Geometry check sheet. Reference: the model listing, model coordinates, mm. A direction names the side the tool comes from. Give positions to 0.01 mm unless a question says otherwise; leave off trailing zeros. Loops run counter-clockwise (first coordinate to the right, second up) from the corner with the lowest first, then second, coordinate; pieces in that order, holes last. Notation, with made-up numbers: (19, 64) - (44, 64) arc R14 cw to (44, 82) - close; hole circle Ø11 at (61.5, 11). An arc over 180 degrees is marked (long way). Use a Markdown table: item, result. Add a question column.
1. Material ranges on L1, parallel to Y at x = -11, z = 24; L2, parallel to Y at x = 30, z = -16; L3, parallel to Z at x = 6.5, y = 6, recorded low to high.
2. Cross-section at C-C on y = 31. Enter the section's corners in (x, z).
3. Cross-section at A-A on y = -19. Enter the section's corners in (x, z), and give its area (3 significant figures).
4. Draft check along X on faces 1 (the flat face through (0, -15, -15)), 2 (the flat face through (0, -50, 0)), 3 (the flat face through (-30, 49, 0)). Enter one of: pulls with the +X half, pulls with the -X half, needs draft (parallel to the pull), parting line crosses it, or undercut.
5. Depth check by flat-ended pin: P1, Ø11, axis at x = 4, z = -23.5, coming from the +Y side; P2, Ø16, axis at y = -9, z = -22, coming from the -X side; P3, Ø8, axis at x = 35.5, z = 39, coming from the -Y side. Enter the tip coordinate at first touch or a pass-through.
6. Cross-section at B-B on x = 0. Enter the section's corners in (y, z), and give its area (3 significant figures).
7. Set-up check for faces 4 (the flat face through (30, 49, 0)), 5 (the flat face through (0, 0, 16)), 6 (the flat face through (0, 49, -7.5)), 7 (the flat face through (5, -15, -22)): record each of +Z, -Z, +X, -X, +Y, -Y from which the full face is reachable in a straight line by a thin tool's end or side.
from build123d import *

# Parameters (mm, degrees)
F0_W     = 60
F0_H     = 15
F1_DEPTH = 100
F3_DEPTH = 30
F4_R     = 50
F4_R_2   = 30
F5_DEPTH = 20
F6_R     = 15
F8_DEPTH = 30


# Not quite as in the source:
# - a feature names something its author has since deleted; it is built from what else it names


with BuildPart() as f1:
    # F0 (on Front) → F1 (new body)
    with BuildSketch(Plane.XZ):
        Rectangle(F0_W, F0_H)
    extrude(amount=-F1_DEPTH)

    # F2 (on face) → F3 (join)
    with BuildSketch(Plane.XZ):
        with BuildLine():
            ThreePointArc((29.0473750966, -7.5), (29.760890888, -3.7801287745), (30, 0))
            ThreePointArc((30, 0), (29.760890888, 3.7801287745), (29.0473750966, 7.5))
            Line((29.0473750966, 7.5), (-29.0473750966, 7.5))
            ThreePointArc((-29.0473750966, 7.5), (-29.760890888, 3.7801287745), (-30, 0))
            ThreePointArc((-30, 0), (-29.760890888, -3.7801287745), (-29.0473750966, -7.5))
            Line((-29.0473750966, -7.5), (29.0473750966, -7.5))
        make_face()
        with BuildLine():
            Line((-29.0473750966, 7.5), (29.0473750966, 7.5))
            ThreePointArc((29.0473750966, 7.5), (0, 30), (-29.0473750966, 7.5))
        make_face()
        with BuildLine():
            ThreePointArc((-29.0473750966, -7.5), (0, -30), (29.0473750966, -7.5))
            Line((29.0473750966, -7.5), (-29.0473750966, -7.5))
        make_face()
    extrude(amount=F3_DEPTH)

    # F4 (on face) → F5 (join)
    with BuildSketch(Plane.XZ.offset(30)):
        Circle(F4_R)
        Circle(F4_R_2, mode=Mode.SUBTRACT)
        Circle(F4_R_2)
    extrude(amount=F5_DEPTH)

    # F6
    f6_edges = [f1.edges().sort_by_distance(p)[0] for p in [
        (-50, -50, 0),
    ]]
    fillet(f6_edges, radius=F6_R)

    # F7 (on face) → F8 (cut)
    with BuildSketch(Plane(origin=(0, 0, 0), x_dir=(-1, 0, 0), z_dir=(0, 1, 0))):
        with BuildLine():
            Line((5, -15), (-5, -15))
            Line((-5, -15), (-5, -29.5803989155))
            ThreePointArc((-5, -29.5803989155), (0, -30), (5, -29.5803989155))
            Line((5, -29.5803989155), (5, -15))
        make_face()
    extrude(amount=-F8_DEPTH, mode=Mode.SUBTRACT)


solid = f1.part
Values found:
| question | item | result |
|---|---|---|
| 1 | L1 | y = -50 to 0 |
| 1 | L2 | y = -50 to -30 |
| 1 | L3 | z = -7.5 to 7.5 |
| 2 | outline | (-30, -7.5) - (30, -7.5) - (30, 7.5) - (-30, 7.5) - close |
| 3 | outline | (-5, -29.58) - (-5, -15) - (5, -15) - (5, -29.58) arc R30 ccw (long way) to start |
| 3 | area | 2,680 mm2 |
| 4 | face 1 | undercut |
| 4 | face 2 | needs draft |
| 4 | face 3 | pulls with the -X half |
| 5 | P1 | stops at y = 0 |
| 5 | P2 | stops at x = -26.53 |
| 5 | P3 | stops at y = -41.02 |
| 6 | outline | (-50, -35) arc R15 ccw to (-35, -50) - (-30, -50) - (-30, -15) - (0, -15) - (0, -7.5) - (100, -7.5) - (100, 7.5) - (0, 7.5) - (0, 30) - (-30, 30) - (-30, 50) - (-35, 50) arc R15 ccw to (-50, 35) - close |
| 6 | area | 4,750 mm2 |
| 7 | face 4 | +Z, -Z, +X, +Y |
| 7 | face 5 | +Z, +X, -X, +Y |
| 7 | face 6 | -Z, +X, -X, +Y |
| 7 | face 7 | -Z, +Y |
